Input: part model. Units: mm. Frame: model coordinates. A direction names the side the tool comes from. Coordinates: 2 decimals unless noted, no trailing zeros. Loops run counter-clockwise (first coordinate to the right, second up) from the corner with the lowest first, then second, coordinate; pieces in that order, holes last. Notation, with made-up numbers: M 85,4.5 L 113,4.5 A19 cw 113,23.5 Z; hole C 45.5,30 d10. An arc over 180 degrees is marked long. Use a Markdown table: item, result. Add a question column.
1. Section A-A on y = 8.75. State how many separate pieces and enclosed holes the cut face has, then the cut area to 3 significant figures.
2. Section D-D on x = 11. Output: boundary loops of the cut face in (y, z).
3. Pin query (flat end, axial travel): pin 1 (3.5 mm diameter, centred on x = 6.5, z = 12.5, fed in from -Y); pin 2 (6.5 mm diameter, centred on x = 23.85, y = 7.28, fed in from +Z); pin 3 (1 mm diameter, centred on x = 22, y = 5, fed in from -Z). Return the tip coordinate at first contact, or that it passes through.
4. Line query: L1, parallel to Z at x = 9, y = 2.75; L2, parallel to Z at x = 10.5, y = 1.5; L3, parallel to X at y = 4.5, z = 3. Output: solid intervals per line, ascending. Write a range as [from, to].
5. Set-up query: faces 5 (the flat face through (8, 2, 10.1)), 6 (the flat face through (26.895, 5.554, 17.268)), 7 (the cylindrical face through (24.63, 3.766, 2.465)), 8 (the cylindrical face through (10.4, 6.7, 5.3)). Return all of +Z, -Z, +X, -X, +Y, -Y with unobstructed straight access to the full face (end or side cutting, diameter ignored); none if empty.
6. Section B-B on z = 17.75. Output: boundary loops of the cut face in (x, y).
7. Draft query along Y for faces 1 (the flat face through (8, 3.9, 8)), 2 (the flat face through (22, 6, 5)), 3 (the flat face through (8, 2, 1.8)), 4 (the flat face through (11, 9.38, 9)). Return one class per face: +Y half, -Y half, draft (parallel to the pull), parting line (faces both ways), or undercut.
Autodesk Inventor part; units mm, degrees
ref_plane "Work Plane1" through (0, 0, 13.37) normal (0, 0, 1) x (1, 0, 0)
ref_plane "YZ Plane" through (0, 0, 0) normal (1, 0, 0) x (0, 1, 0)
ref_plane "XZ Plane" through (0, 0, 0) normal (0, 1, 0) x (-1, 0, 0)
sketch "Sketch1" plane through (0, 0, 0) normal (0, 0, 1) x (1, 0, 0)
  line L0 (0, 0) -> (1.4521, 9.38)
  line L1 (1.4521, 9.38) -> (50.35, 9.38)
  line L2 (50.35, 9.38) -> (50.35, 0)
  line L3 (50.35, 0) -> (0, 0)
  dimension "d7" = 81.2
  dimension "d8" = 50.35
  dimension "d9" = 9.38
extrude "Extrusion1" add sketch "Sketch1" along normal blind 18.5
fillet "Fillet1" radius 2.85 1 edges at (1.4521, 9.38, 9.25)
fillet "Fillet2" radius 1.85 1 edges at (0, 0, 9.25)
sketch "Sketch3" plane through (0, 0, 18.5) normal (0, 0, 1) x (1, 0, 0)
  line L0 (2.1584, 0) -> (50.35, 0)
  line L1 (50.35, 0) -> (50.35, 9.38)
  circle A0 centre (46.18, 4.8) radius 2.25
  point P0 (0, 0)
  dimension "d13" = 4.5
  dimension "d14" = 4.8
  dimension "d15" = 4.17
extrude "Extrusion2" cut sketch "Sketch3" against normal up to next
fillet "Fillet3" radius 4.6 2 edges at (50.35, 9.38, 9.25) (50.35, 0, 9.25)
sketch "Sketch5" plane through (0, 0, 18.5) normal (0, 0, 1) x (1, 0, 0)
  line L0 (45.75, 9.38) -> (3.8948, 9.38)
  arc A0 (29.0413, 9.38) -> (18.6587, 9.38) centre (23.85, 7.28) ccw
  point P0 (50.35, 4.6)
  point P1 (0, 0)
  dimension "d24" = 11.2
  dimension "d25" = 2.1
  dimension "d26" = 26.5
extrude "Extrusion4" add sketch "Sketch5" against normal up to surface (18.5 mm away)
sketch "Sketch6" plane through (0, 0, 18.5) normal (0, 0, 1) x (1, 0, 0)
  arc A0 (29.0413, 9.38) -> (18.6587, 9.38) centre (23.85, 7.28) ccw
  line L0 (27.8915, 7.28) -> (25.8707, 3.78)
  line L1 (25.8707, 3.78) -> (21.8293, 3.78)
  line L2 (21.8293, 3.78) -> (19.8085, 7.28)
  line L3 (19.8085, 7.28) -> (21.8293, 10.78)
  line L4 (21.8293, 10.78) -> (25.8707, 10.78)
  line L5 (25.8707, 10.78) -> (27.8915, 7.28)
  point P0 (0, 0)
  dimension "d29" = 7
extrude "Extrusion5" cut sketch "Sketch6" against normal blind 2.5
sketch "Sketch7" plane through (0, 0, 18.5) normal (0, 0, 1) x (1, 0, 0)
  arc A0 (29.0413, 9.38) -> (18.6587, 9.38) centre (23.85, 7.28) ccw
  circle A1 centre (23.85, 7.28) radius 2
  point P0 (0, 0)
  dimension "d32" = 4
extrude "Extrusion6" cut sketch "Sketch7" against normal up to surface (18.5 mm away)
ref_plane "Work Plane1" through (0, 0, 13.37) normal (0, 0, 1) x (1, 0, 0)
sketch "Sketch8" plane through (0, 0, 13.37) normal (0, 0, 1) x (1, 0, 0)
  circle A0 centre (23.85, 7.28) radius 2
  circle A1 centre (23.85, 7.28) radius 8
  point P0 (0, 0)
  dimension "d36" = 16
extrude "Extrusion7" cut sketch "Sketch8" against normal blind 7
sketch "Sketch9" plane through (0, 0, 18.5) normal (0, 0, 1) x (1, 0, 0)
  line L0 (45.75, 9.38) -> (29.0413, 9.38)
  arc A0 (29.0413, 9.38) -> (18.6587, 9.38) centre (23.85, 7.28) ccw
  circle A1 centre (23.85, 17.79) radius 7.6
  point P0 (0, 0)
  dimension "d39" = 15.2
  dimension "d40" = 8.41
extrude "Extrusion8" cut sketch "Sketch9" against normal blind 4.5
sketch "Sketch10" plane through (0, 0, 0) normal (0, 0, -1) x (-1, 0, 0)
  circle A0 centre (-23.85, 7.28) radius 2
  arc A1 (-18.6587, 9.38) -> (-29.0413, 9.38) centre (-23.85, 7.28) ccw
  circle A2 centre (-23.85, 7.28) radius 3.6
  point P0 (0, 0)
  dimension "d43" = 7.2
extrude "Extrusion9" cut sketch "Sketch10" against normal blind 5
sketch "Sketch11" plane through (3.8948, 9.38, 18.5) normal (0, 1, 0) x (1, 0, 0)
  line L0 (0, 18.5) -> (14.7638, 18.5)
  line L1 (14.7638, 0) -> (0, 0)
  line L2 (3.4252, 13.2) -> (4.2552, 13.2) construction
  line L3 (3.4252, 10.95) -> (4.2552, 10.95)
  line L4 (4.2552, 15.45) -> (3.4252, 15.45)
  arc A0 (3.4252, 15.45) -> (3.4252, 10.95) centre (3.4252, 13.2) ccw
  arc A1 (4.2552, 10.95) -> (4.2552, 15.45) centre (4.2552, 13.2) ccw
  line L5 (3.4252, 4.9) -> (4.2552, 4.9) construction
  line L6 (3.4252, 2.65) -> (4.2552, 2.65)
  line L7 (4.2552, 7.15) -> (3.4252, 7.15)
  arc A2 (3.4252, 7.15) -> (3.4252, 2.65) centre (3.4252, 4.9) ccw
  arc A3 (4.2552, 2.65) -> (4.2552, 7.15) centre (4.2552, 4.9) ccw
  line L8 (46.4552, 0) -> (46.4552, 18.5)
  point P0 (-3.8948, 18.5)
  point P1 (3.8402, 13.2)
  point P2 (3.8402, 4.9)
  dimension "d46" = 4.5
  dimension "d47" = 0.83
  dimension "d48" = 4.9
  dimension "d49" = 5.3
  dimension "d50" = 42.2
extrude "Extrusion10" cut sketch "Sketch11" against normal up to next
sketch "Sketch12" plane through (2.1584, 0, 0) normal (0, -1, 0) x (1, 0, 0)
  arc A0 (5.9916, 3.05) -> (5.9916, 7.55) centre (5.9916, 5.3) ccw
  line L0 (5.9916, 3.05) -> (5.1616, 3.05)
  arc A1 (5.1616, 7.55) -> (5.1616, 3.05) centre (5.1616, 5.3) ccw
  line L1 (5.1616, 7.55) -> (5.9916, 7.55)
  arc A2 (5.9916, 11.35) -> (5.9916, 15.85) centre (5.9916, 13.6) ccw
  line L2 (5.9916, 11.35) -> (5.1616, 11.35)
  arc A3 (5.1616, 15.85) -> (5.1616, 11.35) centre (5.1616, 13.6) ccw
  line L3 (5.1616, 15.85) -> (5.9916, 15.85)
  line L4 (10.033, 13.6) -> (8.0123, 10.1)
  line L5 (8.0123, 10.1) -> (3.9708, 10.1)
  line L6 (3.9708, 10.1) -> (1.9501, 13.6)
  line L7 (1.9501, 13.6) -> (3.9708, 17.1)
  line L8 (3.9708, 17.1) -> (8.0123, 17.1)
  line L9 (8.0123, 17.1) -> (10.033, 13.6)
  line L10 (1.1201, 13.6) -> (3.1408, 17.1)
  line L11 (3.1408, 17.1) -> (7.1823, 17.1)
  line L12 (7.1823, 17.1) -> (9.203, 13.6)
  line L13 (9.203, 13.6) -> (7.1823, 10.1)
  line L14 (7.1823, 10.1) -> (3.1408, 10.1)
  line L15 (3.1408, 10.1) -> (1.1201, 13.6)
  line L16 (10.033, 5.3) -> (8.0123, 1.8)
  line L17 (8.0123, 1.8) -> (3.9708, 1.8)
  line L18 (3.9708, 1.8) -> (1.9501, 5.3)
  line L19 (1.9501, 5.3) -> (3.9708, 8.8)
  line L20 (3.9708, 8.8) -> (8.0123, 8.8)
  line L21 (8.0123, 8.8) -> (10.033, 5.3)
  line L22 (1.1201, 5.3) -> (3.1408, 8.8)
  line L23 (3.1408, 8.8) -> (7.1823, 8.8)
  line L24 (7.1823, 8.8) -> (9.203, 5.3)
  line L25 (9.203, 5.3) -> (7.1823, 1.8)
  line L26 (7.1823, 1.8) -> (3.1408, 1.8)
  line L27 (3.1408, 1.8) -> (1.1201, 5.3)
  point P0 (-2.1584, 0)
  dimension "d53" = 7
extrude "Extrusion11" cut sketch "Sketch12" against normal blind 3.9 contours L0 A1 L1 A0 | L2 A3 L3 A2 | L4 L5 L13 L12 L8 L9 | L5 L6 L7 L8 L12 L13 | L14 L15 L10 L11 L7 L6 | L16 L17 L25 L24 L20 L21 | L17 L18 L19 L20 L24 L25 | L26 L27 L22 L23 L19 L18
properties part number "FelixOriginalBearingHolder"
Answers below:
| question | item | result |
|---|---|---|
| 1 | separate pieces | 2 |
| 1 | enclosed holes | 2 |
| 1 | area | 641 mm² |
| 2 | outline | M 0,0 L 9.38,0 L 9.38,18.5 L 0,18.5 L 0,15.66 L 3.9,15.66 L 3.9,11.54 L 0,11.54 L 0,7.36 L 3.9,7.36 L 3.9,3.24 L 0,3.24 Z |
| 3 | pin 1 | stops at y = 3.9 |
| 3 | pin 2 | stops at z = 16 |
| 3 | pin 3 | stops at z = 5 |
| 4 | L1 | z = [0, 1.8], [8.8, 10.1], [17.1, 18.5] |
| 4 | L2 | z = [0, 2.37], [8.23, 10.67], [16.53, 18.5] |
| 4 | L3 | x = [0.7, 21.56], [26.14, 43.95], [48.41, 50.35] |
| 5 | face 5 | -Y |
| 5 | face 6 | +Z |
| 5 | face 7 | -Z |
| 5 | face 8 | +Y, -Y |
| 6 | outline | M 0.33,2.13 A1.85 ccw 2.16,0 L 45.75,0 A4.6 ccw 50.35,4.6 L 50.35,4.78 A4.6 ccw 45.75,9.38 L 29.04,9.38 A5.6 ccw 27.77,11.28 A7.6 cw 26.03,10.51 L 27.89,7.28 L 25.87,3.78 L 21.83,3.78 L 19.81,7.28 L 21.67,10.51 A7.6 cw 19.93,11.28 A5.6 ccw 18.66,9.38 L 3.89,9.38 A2.85 ccw 1.08,6.97 Z; hole C 46.18,4.8 d4.5 |
| 7 | face 1 | -Y half |
| 7 | face 2 | undercut |
| 7 | face 3 | draft |
| 7 | face 4 | +Y half |
